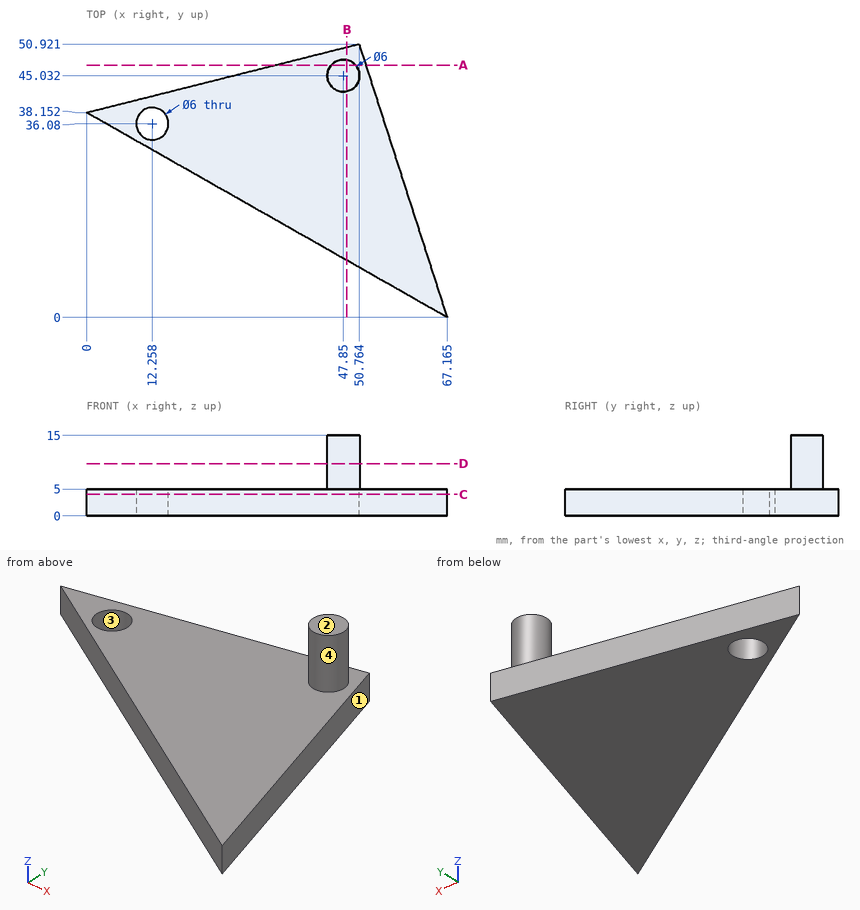
Part print with two shaded views. Sizes in mm from the minimum x, y, z corner. Give positions to 0.01 mm unless a question says otherwise; leave off trailing zeros. Order: outer loops, then holes, each group sorted by start corner. A loop starts at its lowest first (then second) coordinate and runs counter-clockwise, first axis right, second up. Notation, with made-up numbers: M 6.25,32 L 65.25,32 A16 cw 65.25,50 Z; hole C -7,-28.5 d8. An arc over 180 degrees is marked long. Use one line per item in the form item = value.
1) Saw through at B-B (x = 48.5). Give the cut face in (y, z).
Calculated:
outline = M 10.6,0 L 50.35,0 L 50.35,5 L 47.96,5 L 47.96,15 L 42.1,15 L 42.1,5 L 10.6,5 Z
2) Probe probe 1 along Z at (x, y) = (38, 47); probe 2 along X at (y, z) = (33.5, 1) (1 decimal); probe 3 along X at (y, z) = (36, 2.25) (1 decimal). List the from-to ranges inside material, lowest first.
Calculated:
probe_1 = 0 to 5
probe_2 = 8.2 to 10.7, 13.8 to 56.4
probe_3 = 3.8 to 9.3, 15.3 to 55.6
3) Drop flat-ended pins along their axis: pin 1 (4 mm diameter, centred on y = 18, z = 6, fed in from +X) (1 decimal); pin 2 (2 mm diameter, centred on y = 9.5, z = 3.5, fed in from +X); pin 3 (4 mm diameter, centred on y = 5.5, z = 2.5, fed in from +X); pin 4 (3.5 mm diameter, centred on x = 12.26, y = 36.08, fed in from -Z). Give the stop position or say it passes through.
Calculated:
pin_1 = 61.9
pin_2 = 64.43
pin_3 = 66.04
pin_4 = through
4) Saw through at C-C (z = 4). Give the cut face in (x, y) (1 decimal), plus the area to 3 significant figures.
Calculated:
outline = M 0,38.2 L 67.2,0 L 50.8,50.9 Z; hole C 12.3,36.1 d6
area = 1,370 mm2
5) Saw through at A-A (y = 47). Give the cut face in (x, z) (1 decimal).
Calculated:
outline = M 35.2,0 L 52,0 L 52,5 L 50.1,5 L 50.1,15 L 45.6,15 L 45.6,5 L 35.2,5 Z
6) Saw through at D-D (z = 9.75). Give the cut face in (x, y).
Calculated:
outline = C 47.85,45.03 d6
7) Two-plate mould, pull along Y, no slides. Class the marked faces 1, 2, 3 and 4: released by +Y, released by -Y, zero draft, split by the parting line, or undercut.
Calculated:
face_1 = released by +Y
face_2 = zero draft
face_3 = undercut
face_4 = split by the parting line
